Can you work these out from the model? Positions are in its coordinate system, mm. Face numbers are marked on the shaded views. A direction names the side the tool comes from. Round coordinates to 2 decimals unless told otherwise and drop trailing zeros. Write each loop counter-clockwise with the first axis right and the second up, starting at its lowest first coordinate (ties: lowest second). Pieces come first, ordered by that corner, then holes. Notation, with made-up numbers: (25.5, 57.25) -> (43.5, 57.25) arc R21 cw to (43.5, 63.25) -> close; hole circle Ø11 at (-9, -1.5). An arc over 180 degrees is marked (long way). Write item = value, one per line. Start each with the question number.
1) Imagine slicing it at D-D, the plane x = 0. State how many separate pieces and enclosed holes the cut face has, then the cut area to 3 significant figures.
2) Imagine slicing it at B-B, the plane z = -12. Please give me the cut outline in (x, y), then the cut area to 4 significant figures.
3) I'm going to push flat-ended pins straight in: pin 1 (6 mm diameter, centred on x = -7, y = 18.5, fed in from -Z); pin 2 (3 mm diameter, centred on x = 0, z = -12, fed in from +Y); pin 3 (5 mm diameter, centred on x = 5, y = 18.5, fed in from +Z); pin 4 (6 mm diameter, centred on x = 1.5, y = 7.5, fed in from +Z). Where does each tip first touch, or does it pass through?
4) For the marked faces 1, 2 and 3, which set-ups out of +Z, -Z, +X, -X, +Y, -Y let a thin tool reach every point of the face, with its end or its side?
5) If I drill on line 1 (X direction, y = 3.75, z = 12); line 2 (Z direction, x = -0.25, y = 22.25); line 3 (X direction, y = 0.8, z = -12), over which ranges is the centre line in solid material (lowest first)?
6) Imagine slicing it at A-A, the plane z = 0. Please give me the cut outline in (x, y).
7) Imagine slicing it at C-C, the plane y = 11.5. Please give me the cut outline in (x, z), then the cut area to 3 significant figures.
8) Thinking about a two-plate mould opening in Z: for the marked faces 4, 5 and 6, which applies, +Z half, -Z half, draft (parallel to the pull), parting line (faces both ways), or undercut?
from build123d import *

# Parameters (mm, degrees)
SKETCH1_R           = 16
BOSS_EXTRUDE1_DEPTH = 5
CUT_EXTRUDE1_DEPTH  = 5
SKETCH3_R           = 7.5
BOSS_EXTRUDE2_DEPTH = 18
SKETCH4_R           = 4
CUT_EXTRUDE2_DEPTH  = 23
SKETCH5_R           = 1.75
CUT_EXTRUDE3_DEPTH  = 5
SKETCH6_R           = 3
CUT_EXTRUDE4_DEPTH  = 3
CHAMFER1_SIZE       = 0.25


with BuildPart() as part:
    # Sketch1 → Boss-Extrude1 (new body)
    with BuildSketch(Plane(origin=(0, 0, 0), x_dir=(1, 0, 0), z_dir=(0, 1, 0))):
        with Locations(Location((0, 0, 0), (0, 0, 270))):
            Circle(SKETCH1_R)
    extrude(amount=BOSS_EXTRUDE1_DEPTH)

    # Sketch2 → Cut-Extrude1 (cut)
    with BuildSketch(Plane(origin=(0, 0, 0), x_dir=(1, 0, 0), z_dir=(0, 1, 0))):
        with BuildLine():
            Line((-10, 12.489995997), (-10, -12.489995997))
            ThreePointArc((-10, -12.489995997), (-16, 0), (-10, 12.489995997))
        make_face()
        with BuildLine():
            Line((10, 12.489995997), (10, -12.489995997))
            ThreePointArc((10, -12.489995997), (16, 0), (10, 12.489995997))
        make_face()
    extrude(amount=CUT_EXTRUDE1_DEPTH, mode=Mode.SUBTRACT)

    # Sketch3 → Boss-Extrude2 (add)
    with BuildSketch(Plane(origin=(0, 5, 0), x_dir=(1, 0, 0), z_dir=(0, 1, 0))):
        with Locations(Location((0, 0, 0), (0, 0, 270))):
            Circle(SKETCH3_R)
    extrude(amount=BOSS_EXTRUDE2_DEPTH)

    # Sketch4 → Cut-Extrude2 (cut)
    with BuildSketch(Plane(origin=(0, 23, 0), x_dir=(1, 0, 0), z_dir=(0, 1, 0))):
        with Locations(Location((0, 0, 0), (0, 0, 270))):
            Circle(SKETCH4_R)
    extrude(amount=-CUT_EXTRUDE2_DEPTH, mode=Mode.SUBTRACT)

    # Sketch5 → Cut-Extrude3 (cut)
    with BuildSketch(Plane(origin=(0, 5, 0), x_dir=(1, 0, 0), z_dir=(0, 1, 0))):
        with Locations(Location((0, 12, 0), (0, 0, 270))):
            Circle(SKETCH5_R)
        with Locations(Location((0, -12, 0), (0, 0, 270))):
            Circle(SKETCH5_R)
    extrude(amount=-CUT_EXTRUDE3_DEPTH, mode=Mode.SUBTRACT)

    # Sketch6 → Cut-Extrude4 (cut)
    with BuildSketch(Plane.XZ):
        with Locations(Location((0, 12, 0), (0, 0, 270))):
            Circle(SKETCH6_R)
        with Locations(Location((0, -12, 0), (0, 0, 270))):
            Circle(SKETCH6_R)
    extrude(amount=-CUT_EXTRUDE4_DEPTH, mode=Mode.SUBTRACT)

    # Chamfer1
    chamfer1_edges = [part.edges().sort_by_distance(p)[0] for p in [
        (0, 0, -16),
        (0, 5, -16),
        (10, 0, 0),
        (10, 5, 0),
        (0, 23, -7.5),
        (0, 0, -4),
        (0, 23, -4),
        (0, 5, -13.75),
        (0, 5, 10.25),
        (0, 0, 15),
        (0, 0, -9),
        (0, 0, 16),
        (0, 5, 16),
        (-10, 0, 0),
        (-10, 5, 0),
    ]]
    chamfer(chamfer1_edges, length=CHAMFER1_SIZE)


solid = part.part
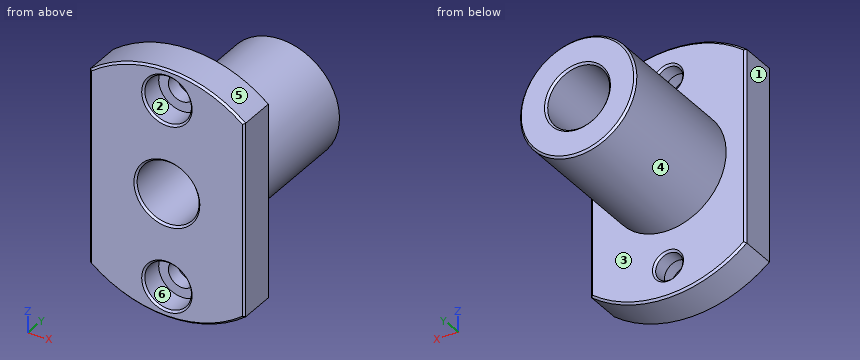
Reported:
q1.separate_pieces = 4
q1.enclosed_holes = 0
q1.area = 195 mm²
q2.outline = (-10, 0.25) -> (-9.75, 0) -> (-3.25, 0) -> (-3, 0.25) -> (-3, 3) -> (-1.75, 3) -> (-1.75, 4.75) -> (-2, 5) -> (-9.75, 5) -> (-10, 4.75) -> close; (1.75, 3) -> (3, 3) -> (3, 0.25) -> (3.25, 0) -> (9.75, 0) -> (10, 0.25) -> (10, 4.75) -> (9.75, 5) -> (2, 5) -> (1.75, 4.75) -> close
q2.area = 74.75 mm²
q3.pin_1 = -6.34
q3.pin_2 = through
q3.pin_3 = 7.07
q3.pin_4 = 16
q4.face_1 = +Z, -Z, -X, +Y, -Y
q4.face_2 = -Y
q4.face_3 = +Y
q5.line_1 = -10 to -1.75, 1.75 to 10
q5.line_2 = -7.5 to -3.99, 3.99 to 7.5
q5.line_3 = -10 to -3, 3 to 10
q6.outline = (-10, 0.25) -> (-9.75, 0) -> (-4.25, 0) -> (-4, 0.25) -> (-4, 22.75) -> (-4.25, 23) -> (-7.25, 23) -> (-7.5, 22.75) -> (-7.5, 5) -> (-9.75, 5) -> (-10, 4.75) -> close; (4, 0.25) -> (4.25, 0) -> (9.75, 0) -> (10, 0.25) -> (10, 4.75) -> (9.75, 5) -> (7.5, 5) -> (7.5, 22.75) -> (7.25, 23) -> (4.25, 23) -> (4, 22.75) -> close
q7.outline = circle Ø15 at (0, 0); hole circle Ø8 at (0, 0)
q7.area = 126 mm²
q8.face_4 = parting line
q8.face_5 = +Z half
q8.face_6 = undercut
